from build123d import *

# Parameters (mm, degrees)
F1_DEPTH = 25


with BuildPart() as f1:
    # F0 (on Top) → F1 (new body)
    with BuildSketch(Plane.XY):
        with BuildLine():
            Line((-22.786474, -11.536708), (-7.983426, -11.536708))
            ThreePointArc((-7.983426, -11.536708), (-6.215659, -10.804475), (-5.483426, -9.036708))
            Line((-5.483426, -9.036708), (-5.483426, -0.607649))
            Line((-5.483426, -0.607649), (-1.672428, -4.450142))
            Line((-1.672428, -4.450142), (2.044082, -0.607649))
            Line((2.044082, -0.607649), (2.044082, -11.536708))
            Line((2.044082, -11.536708), (10.075524, -11.536708))
            Line((10.075524, -11.536708), (10.075524, -4.576126))
            Line((10.075524, -4.576126), (14.862892, -11.536708))
            Line((14.862892, -11.536708), (19.524276, -11.536708))
            ThreePointArc((19.524276, -11.536708), (21.645597, -10.658028), (22.524276, -8.536708))
            Line((22.524276, -8.536708), (22.524276, 10.158991))
            Line((22.524276, 10.158991), (14.685626, 10.158991))
            Line((14.685626, 10.158991), (14.685626, 3.457541))
            Line((14.685626, 3.457541), (10.931709, 9.008034))
            ThreePointArc((10.931709, 9.008034), (9.965858, 9.877737), (8.705565, 10.195408))
            Line((8.705565, 10.195408), (-20.13615, 10.306249))
            ThreePointArc((-20.13615, 10.306249), (-22.311759, 9.415733), (-22.786474, 7.113356))
            Line((-22.786474, 7.113356), (-22.786474, 7.220973))
            Line((-22.786474, 7.220973), (-19.752085, 7.220973))
            Line((-19.752085, 7.220973), (-19.752085, 7.267032))
            ThreePointArc((-19.752085, 7.267032), (-19.401118, 8.114342), (-18.553809, 8.465309))
            Line((-18.553809, 8.465309), (-14.427898, 8.465309))
            ThreePointArc((-14.427898, 8.465309), (-13.463502, 8.065843), (-13.064036, 7.101447))
            Line((-13.064036, 7.101447), (-13.064036, 6.980661))
            ThreePointArc((-13.064036, 6.980661), (-13.44803, 6.053618), (-14.375072, 5.669625))
            Line((-14.375072, 5.669625), (-17.249033, 5.669625))
            Line((-17.249033, 5.669625), (-17.249033, 4.13342))
            Line((-17.249033, 4.13342), (-14.804287, 4.13342))
            ThreePointArc((-14.804287, 4.13342), (-13.890238, 3.755928), (-13.508925, 2.843465))
            Line((-13.508925, 2.843465), (-13.506027, 2.150697))
            ThreePointArc((-13.506027, 2.150697), (-13.833554, 1.350526), (-14.630957, 1.016315))
            Line((-14.630957, 1.016315), (-18.474126, 1.000238))
            ThreePointArc((-18.474126, 1.000238), (-19.391586, 1.390063), (-19.740027, 2.324025))
            Line((-19.740027, 2.324025), (-19.712353, 2.889719))
            Line((-19.712353, 2.889719), (-22.861291, 2.917016))
            Line((-22.861291, 2.917016), (-22.861291, 2.005195))
            ThreePointArc((-22.861291, 2.005195), (-22.129058, 0.237428), (-20.361291, -0.494805))
            Line((-20.361291, -0.494805), (-22.861291, -0.494805))
            Line((-22.861291, -0.494805), (-22.786474, -9.606927))
            Line((-22.786474, -9.606927), (-22.786474, -11.536708))
        make_face()
        with BuildLine():
            Line((-19.634925, -9.606927), (-19.634925, -2.168437))
            Line((-19.634925, -2.168437), (-15.943606, -2.168437))
            ThreePointArc((-15.943606, -2.168437), (-14.175839, -2.90067), (-13.443606, -4.668437))
            Line((-13.443606, -4.668437), (-13.443606, -7.106927))
            ThreePointArc((-13.443606, -7.106927), (-14.175839, -8.874694), (-15.943606, -9.606927))
            Line((-15.943606, -9.606927), (-19.634925, -9.606927))
        make_face(mode=Mode.SUBTRACT)
    extrude(amount=F1_DEPTH)


solid = f1.part
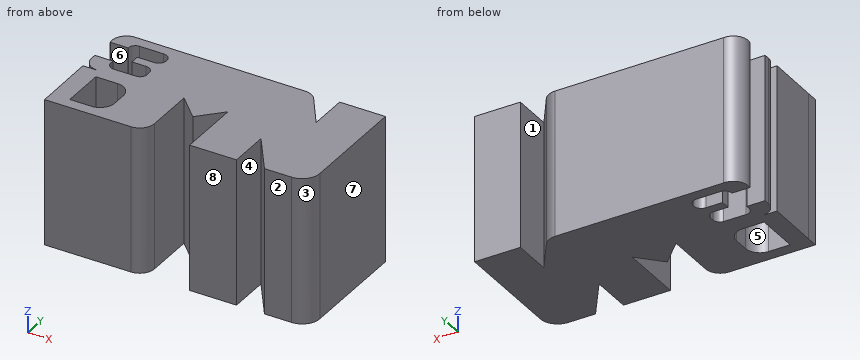
Can you work these out from the model? Positions are in its coordinate system, mm. Face numbers are marked on the shaded views. A direction names the side the tool comes from. Give positions to 0.01 mm unless a question says otherwise; leave off trailing zeros. Write each loop counter-clockwise with the first axis right and the second up, starting at its lowest first coordinate (ties: lowest second). Pieces come first, ordered by that corner, then holes. Notation, with made-up numbers: (-38.5, 80) -> (19.5, 80) arc R19 cw to (19.5, 107) -> close; hole circle Ø1 at (20, -33.5). An arc over 180 degrees is marked (long way). Answer as a JSON object with one key per item and string values. Group by question number.
Item 1: Suppose I cut it at C-C (x = -4.5). Please give me the cut outline in (y, z), plus the area to 3 significant figures.
Item 2: Suppose I cut it at B-B (y = 1.5). Please give me the cut outline in (x, z), plus the area to 3 significant figures.
Item 3: For the marked faces 1, 2, 3, 4 and 5, which set-ups out of +Z, -Z, +X, -X, +Y, -Y let a thin tool reach every point of the face, with its end or its side?
Item 4: I'm going to push flat-ended pins straight in: P1, Ø6, axis at x = 0.5, y = -5, coming from the +Z side; P2, Ø0.9, axis at x = -16.5, z = 18, coming from the +Y side; P3, Ø6.5, axis at x = 19, z = 7, coming from the +Y side; P4, Ø5.5, axis at y = -4, z = 9, coming from the -X side. Where does each tip first touch, or does it pass through?
Item 5: We'd pull the mould along Y, two halves only. Please class the marked faces 6, 7 and 8: +Y half, -Y half, draft (parallel to the pull), parting line (faces both ways), or undercut.
Item 6: Suppose I cut it at A-A (y = 6.25). Please give me the cut outline in (x, z).
Item 7: Please list where these lines run through material, in increasing order: line 1 (Y direction, x = -18, z = 20.5); line 2 (X direction, y = -4, z = 17); line 3 (X direction, y = -10, z = 4.75). Write a range as [from, to].
Findings:
{
 "1": {"outline": "(-1.6, 0) -> (10.25, 0) -> (10.25, 25) -> (-1.6, 25) -> close", "area": "296 mm²"},
 "2": {"outline": "(-22.81, 0) -> (-19.49, 0) -> (-19.49, 25) -> (-22.81, 25) -> close; (-13.71, 0) -> (22.52, 0) -> (22.52, 25) -> (-13.71, 25) -> close", "area": "989 mm²"},
 "3": {"face 1": "+Z, -Z, +Y", "face 2": "+Z, -Z, +X, -X, -Y", "face 3": "+Z, -Z, +X, -Y", "face 4": "+Z, -Z, -Y", "face 5": "+Z, -Z"},
 "4": {"P1": "stops at z = 25", "P2": "stops at y = 10.29", "P3": "stops at y = 10.16", "P4": "stops at x = -22.86"},
 "5": {"face 6": "undercut", "face 7": "draft", "face 8": "-Y half"},
 "6": {"outline": "(-13.29, 0) -> (12.8, 0) -> (12.8, 25) -> (-13.29, 25) -> close; (14.69, 0) -> (22.52, 0) -> (22.52, 25) -> (14.69, 25) -> close"},
 "7": {"line 1": "y = [-11.54, -9.61], [-2.17, 1], [8.47, 10.3]", "line 2": "x = [-22.83, -19.63], [-13.53, -5.48], [-2.12, -1.24], [2.04, 22.52]", "line 3": "x = [-22.79, -5.68], [2.04, 10.08], [13.81, 22.14]"}
}
